CAD build for the part. Positions are in the model's coordinates, mm. A direction names the side the tool comes from. Coordinates: 2 decimals unless noted, no trailing zeros. Loops run counter-clockwise (first coordinate to the right, second up) from the corner with the lowest first, then second, coordinate; pieces in that order, holes last. Notation, with made-up numbers: (24.5, 61.25) -> (53.5, 61.25) arc R35 cw to (53.5, 96.25) -> close; hole circle Ø11 at (72.25, 51). An arc over 180 degrees is marked (long way). Return JSON: item names as keys, results as strings. Group by question number.
(1) Tool access for faces 1 (the face through (3.55, 119.83, 10.41)), 2 (the face through (-4, 108.396, 10)), 3 (the face through (-11, 130.396, 10)): list every direction of +Z, -Z, +X, -X, +Y, -Y with a clear straight run to the whole face (end or side of a thin tool).
(2) Mould opens along X. For faces 4 (the face through (3.549, 113.486, 16.664)), 5 (the face through (-7.2, 119, 10)), 6 (the face through (7, 111, 12)) say: pulls with the +X half, pulls with the -X half, needs draft (parallel to the pull), parting line crosses it, or undercut.
(3) Saw through at B-B on z = 15.5. Give the number of separate pieces and of enclosed holes in the cut face, then the cut area to 3 significant figures.
(4) Flat gauge pins, fed straight in: pin 1 Ø6 at (y, z) = (113.4, 14.62) entering from -X; pin 2 Ø6 at (y, z) = (124, 2) entering from +X; pin 3 Ø6 at (y, z) = (124.5, 5.5) entering from -X. Where does each tip first touch, or does it go through?
(5) Probe L1, parallel to X at y = 121, z = 12.75; L2, parallel to X at y = 117.5, z = 18; L3, parallel to Z at x = -31, y = 113.5. List the from-to ranges inside material, lowest first.
(6) Saw through at A-A on x = -12. Write the cut outline in (y, z).
```python
from build123d import *

# Parameters (mm, degrees)
BOSS_EXTRUDE1_DEPTH = 20
SKETCH2_R           = 53
SKETCH2_R_2         = 2.05
CUT_EXTRUDE1_DEPTH  = 14.2
SKETCH4_R           = 1.85
CUT_EXTRUDE2_DEPTH  = 56


with BuildPart() as part:
    # Sketch1 → Boss-Extrude1 (new body)
    with BuildSketch(Plane.XY):
        with BuildLine():
            Line((0, 130.395512055), (0, 108.395512055))
            Line((0, 108.395512055), (-7.2, 108.395512055))
            Line((-7.2, 108.395512055), (-7.2, 130.395512055))
            Line((-7.2, 130.395512055), (-14.2, 130.395512055))
            add(Edge.make_bspline(
                [(-14.2, 130.395512055), (-23.530576474, 124.205565192), (-38.446210931, 100.318296321), (-66.691471381, 105.395512055), (-83, 105.395512055)],
                knots=[0, 0, 0, 0, 0.267223526, 1, 1, 1, 1], degree=3))
            Line((-83, 105.395512055), (-83, 98.395512055))
            Line((-83, 98.395512055), (7, 98.395512055))
            Line((7, 98.395512055), (7, 130.395512055))
            Line((7, 130.395512055), (0, 130.395512055))
        make_face()
    extrude(amount=BOSS_EXTRUDE1_DEPTH)

    # Sketch2 → Cut-Extrude1 (cut)
    with BuildSketch(Plane(origin=(7, 0, 0), x_dir=(0, 0, -1), z_dir=(1, 0, 0))):
        with Locations((28.164207495, 156.175472317)):
            Circle(SKETCH2_R)
        with Locations((-14.615752767, 113.395512055)):
            Circle(SKETCH2_R_2)
    extrude(amount=-CUT_EXTRUDE1_DEPTH, mode=Mode.SUBTRACT)

    # Sketch4 → Cut-Extrude2 (cut)
    with BuildSketch(Plane(origin=(7, 0, 0), x_dir=(0, 0, -1), z_dir=(1, 0, 0))):
        with Locations((-14.615752767, 113.395512055)):
            Circle(SKETCH4_R)
    extrude(amount=-CUT_EXTRUDE2_DEPTH, mode=Mode.SUBTRACT)


solid = part.part
```
Geometry results:
{
 "1": {"face 1": "-Z, +X, +Y", "face 2": "+Z, -Z, +Y", "face 3": "+Z, -Z, +X, -X, +Y"},
 "2": {"face 4": "needs draft", "face 5": "undercut", "face 6": "pulls with the +X half"},
 "3": {"separate pieces": "3", "enclosed holes": "0", "area": "1,220 mm²"},
 "4": {"pin 1": "x = -36.73", "pin 2": "x = -7.2", "pin 3": "x = -24.73"},
 "5": {"L1": "-25.21 to -7.2, 0 to 7", "L2": "-28.46 to -7.2, 0 to 7", "L3": "0 to 12.77, 16.46 to 20"},
 "6": {"outline": "(98.4, 0) -> (130.4, 0) -> (130.4, 20) -> (98.4, 20) -> close; hole circle Ø3.7 at (113.4, 14.62)"}
}
